For this review, use the dimensioned drawing (mm, ordinates from the lowest corner) and the shaded views. A direction names the side the tool comes from. Round coordinates to 2 decimals unless told otherwise and drop trailing zeros. Write each loop counter-clockwise with the first axis right and the second up, starting at its lowest first coordinate (ties: lowest second). Pieces come first, ordered by that corner, then holes. Notation, with made-up numbers: (32, -24.5) -> (79, -24.5) arc R15 cw to (79, -3.5) -> close; hole circle Ø9 at (31.5, -36). An arc over 180 degrees is marked (long way). Answer in a Markdown table with one row per item. Add a question column.
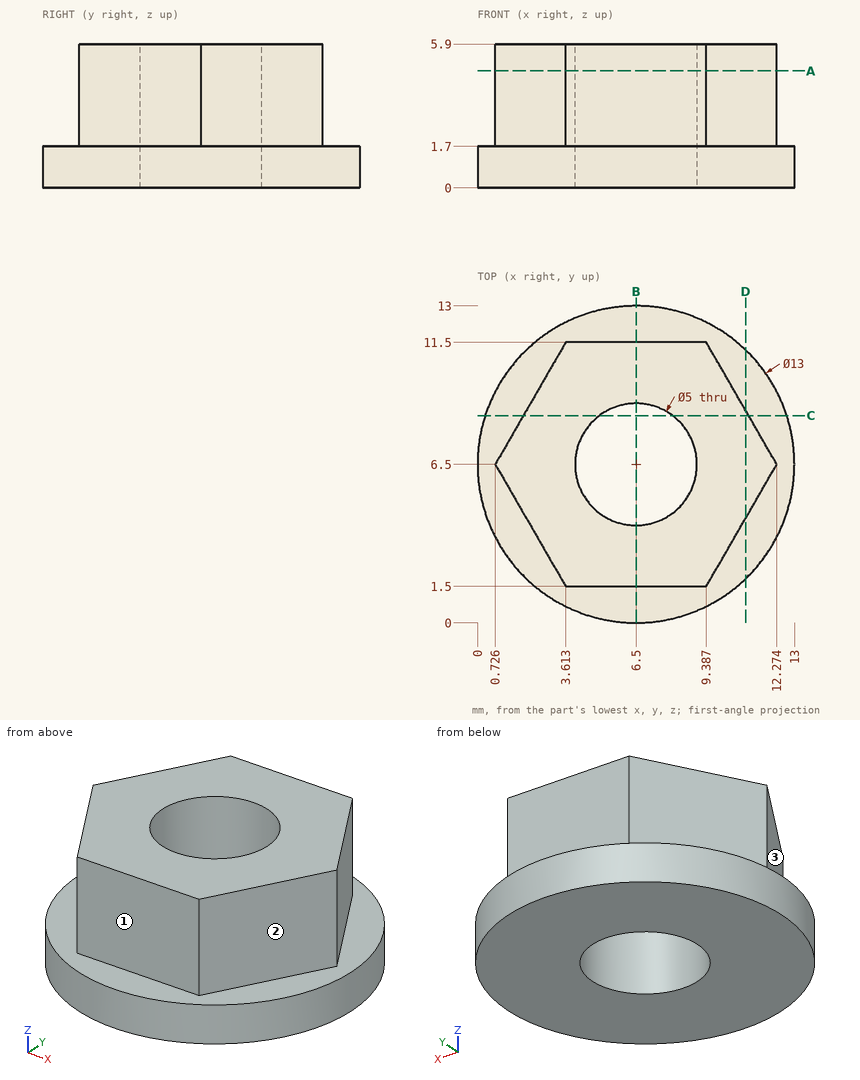
1. We need section D-D (x = 11). Write out the cut boundary in (y, z) (1 decimal).
2. We need section B-B (x = 6.5). Write out the cut boundary in (y, z), plus the area to 3 significant figures.
3. For L1, parallel to Y at x = 6.5, z = 2.75; L2, parallel to Y at x = 6.5, z = 1.25; L3, parallel to Z at x = 8.75, y = 12.25, list the stretches that pass through material, from the lowest coordinate up. Write a range as [from, to].
4. Tool access review of the marked faces 1, 2 and 3: name each direction out of +Z, -Z, +X, -X, +Y, -Y from which nothing blocks a thin tool from reaching the whole face with its end or side.
5. We need section A-A (z = 4.8). Write out the cut boundary in (x, y).
6. We need section C-C (y = 8.5). Write out the cut boundary in (x, z) (1 decimal).
7. Clearance check with flat-ended pins moving along their axes: pin 1 Ø1.5 at (x, y) = (6, 4.5) entering from +Z; pin 2 Ø1.3 at (x, z) = (6.5, 3.5) entering from +Y. State where each tip first meets the part, or that it passes through.
Response:
| question | item | result |
|---|---|---|
| 1 | outline | (1.8, 0) -> (11.2, 0) -> (11.2, 1.7) -> (8.7, 1.7) -> (8.7, 5.9) -> (4.3, 5.9) -> (4.3, 1.7) -> (1.8, 1.7) -> close |
| 2 | outline | (0, 0) -> (4, 0) -> (4, 5.9) -> (1.5, 5.9) -> (1.5, 1.7) -> (0, 1.7) -> close; (9, 0) -> (13, 0) -> (13, 1.7) -> (11.5, 1.7) -> (11.5, 5.9) -> (9, 5.9) -> close |
| 2 | area | 34.6 mm2 |
| 3 | L1 | [1.5, 4], [9, 11.5] |
| 3 | L2 | [0, 4], [9, 13] |
| 3 | L3 | [0, 1.7] |
| 4 | face 1 | +Z, +X, -X, -Y |
| 4 | face 2 | +Z, +X, -Y |
| 4 | face 3 | +Z, -X, -Y |
| 5 | outline | (0.73, 6.5) -> (3.61, 1.5) -> (9.39, 1.5) -> (12.27, 6.5) -> (9.39, 11.5) -> (3.61, 11.5) -> close; hole circle Ø5 at (6.5, 6.5) |
| 6 | outline | (0.3, 0) -> (5, 0) -> (5, 5.9) -> (1.9, 5.9) -> (1.9, 1.7) -> (0.3, 1.7) -> close; (8, 0) -> (12.7, 0) -> (12.7, 1.7) -> (11.1, 1.7) -> (11.1, 5.9) -> (8, 5.9) -> close |
| 7 | pin 1 | z = 5.9 |
| 7 | pin 2 | y = 11.5 |
